```python
from build123d import *

# Parameters (mm, degrees)
F0_W     = 304.8
F0_H     = 30.48
F1_DEPTH = 152.4
F2_W     = 25
F2_H     = 20
F3_DEPTH = 70
F5_DEPTH = 152.4


# Not quite as in the source:
# - the program builds the solid bodies; features that only make, move or delete a surface that nothing else refers to are left out


with BuildPart() as f1:
    # F0 (on Front) → F1 (new body)
    with BuildSketch(Plane.XZ):
        Rectangle(F0_W, F0_H)
    extrude(amount=F1_DEPTH)

    # F2 (on face) → F3 (join)
    with BuildSketch(Plane.XY.offset(15.24)):
        with Locations((-139.9, -10)):
            Rectangle(F2_W, F2_H)
        with Locations((-139.9, -142.4)):
            Rectangle(F2_W, F2_H)
        with Locations((139.9, -10)):
            Rectangle(F2_W, F2_H)
        with Locations((139.9, -142.4)):
            Rectangle(F2_W, F2_H)
    extrude(amount=F3_DEPTH)

    # F4 (on Front) → F5 (join)
    with BuildSketch(Plane.XZ):
        with BuildLine():
            Line((124.2321878223, -65.5579566956), (151.5389296347, -62.7254612585))
            ThreePointArc((151.5389296347, -62.7254612585), (-3.7822030549, 7.8738857172), (-157.7844321728, -65.5579566956))
            Line((-157.7844321728, -65.5579566956), (-124.8654021339, -65.5579566956))
            ThreePointArc((-124.8654021339, -65.5579566956), (-0.3166071558, -14.6454567478), (124.2321878223, -65.5579566956))
        make_face()
    extrude(amount=F5_DEPTH)


solid = f1.part
```
Geometry check sheet. Reference: the model listing, model coordinates, mm. A direction names the side the tool comes from. Coordinates: 2 decimals unless noted, no trailing zeros. Write each loop counter-clockwise with the first axis right and the second up, starting at its lowest first coordinate (ties: lowest second). Pieces come first, ordered by that corner, then holes. Notation, with made-up numbers: M 35.25,-15 L 54.25,-15 A23 ccw 54.25,2 Z; hole C 12,45 d7. An arc over 180 degrees is marked long. One line per item, written item: value. Start each with the question number.
(1) Release check for a two-part mould opening along Z. For faces 4 (the face through (-140, -10, 85.24)), 5 (the face through (127.4, -143, 50)), 6 (the face through (-128.86, -75.13, -36.95)) record: released by +Z, released by -Z, zero draft, split by the parting line, or undercut.
(2) Depth check by flat-ended pin: pin 1 (12 mm diameter, centred on x = -102.5, y = -71, fed in from -Z); pin 2 (22 mm diameter, centred on y = -14.5, z = 56, fed in from -X); pin 3 (1 mm diameter, centred on y = -21, z = -45, fed in from -X); pin 4 (5 mm diameter, centred on x = 63, z = 19, fed in from -Y). Enter the tip coordinate at first touch or a pass-through.
(3) Sectioned sample at C-C, the plane x = 132. Enter the section's corners in (y, z), and give its area (3 significant figures).
(4) Sectioned sample at D-D, the plane x = 5. Enter the section's corners in (y, z), and give its area (3 significant figures).
(5) Sectioned sample at A-A, the plane z = 35. Enter the section's corners in (x, y), and give its area (3 significant figures).
(6) Sectioned sample at B-B, the plane y = -98. Enter the section's corners in (x, z).
(7) Tool access check on faces 1 (the face through (122, -75, -15.24)), 2 (the face through (140, -132.4, 50)), 3 (the face through (127.4, -10, 50)). Record the directions out of +Z, -Z, +X, -X, +Y, -Y that give a thin tool (end or side, any length) a straight path to the whole face; none if there is none.
(8) Scan lines: line 1 along X through (y, z) = (-143.5, 53); line 2 along X through (y, z) = (-67.5, 0.5); line 3 along X through (y, z) = (-73, -27). Record each from-to range of solid material in increasing order. Write a range as [from, to].
Filled sheet:
1. face 4: released by +Z
1. face 5: zero draft
1. face 6: undercut
2. pin 1: z = -51.35
2. pin 2: x = -152.4
2. pin 3: x = -138.78
2. pin 4: through
3. outline: M -152.4,-64.75 L 0,-64.75 L 0,-42.87 L -152.4,-42.87 Z; M -152.4,-15.24 L 0,-15.24 L 0,85.24 L -20,85.24 L -20,15.24 L -132.4,15.24 L -132.4,85.24 L -152.4,85.24 Z
3. area: 10,800 mm²
4. outline: M -152.4,-15.24 L 0,-15.24 L 0,15.24 L -152.4,15.24 Z
4. area: 4,650 mm²
5. outline: M -152.4,-152.4 L -127.4,-152.4 L -127.4,-132.4 L -152.4,-132.4 Z; M -152.4,-20 L -127.4,-20 L -127.4,0 L -152.4,0 Z; M 127.4,-152.4 L 152.4,-152.4 L 152.4,-132.4 L 127.4,-132.4 Z; M 127.4,-20 L 152.4,-20 L 152.4,0 L 127.4,0 Z
5. area: 2,000 mm²
6. outline: M -157.78,-65.56 L -124.87,-65.56 A177.8 cw -14.84,-15.24 L 14.21,-15.24 A177.8 cw 124.23,-65.56 L 151.54,-62.73 A202.09 ccw 91.94,-15.24 L 152.4,-15.24 L 152.4,15.24 L -152.4,15.24 L -152.4,-15.24 L -95.8,-15.24 A202.09 ccw Z
7. face 1: +X, +Y, -Y
7. face 2: +Z, +X, -X
7. face 3: +Z, +Y, -Y
8. line 1: [-152.4, -127.4], [127.4, 152.4]
8. line 2: [-152.4, 152.4]
8. line 3: [-115.43, -65.44], [64.8, 111.57]
